Part model, mm, in its own coordinate system. Round coordinates to 2 decimals unless told otherwise and drop trailing zeros. Loops run counter-clockwise (first coordinate to the right, second up) from the corner with the lowest first, then second, coordinate; pieces in that order, holes last. Notation, with made-up numbers: (-5.75, 40) - (14.25, 40) arc R24 cw to (14.25, 51) - close; hole circle Ø9 at (-39, -19). An arc over 180 degrees is marked (long way). Write each question's results on one line, items separated by ' | '. Start each with the question number.
(1) Mould opens along Y. For faces 1 (the face through (45, 0, 1)), 2 (the face through (0, -27, 1)), 3 (the face through (-42.49, 24.13, 0.81)) say: released by +Y, released by -Y, zero draft, split by the parting line, or undercut.
(2) Flat gauge pin, fed straight in: P1, Ø2.5, axis at x = -41.3, y = -24, coming from the +Z side. Where does the tip first touch, or does it go through?
(3) Cut at A-A, the plane y = -24. List the corners of the cut face in (x, z), then the cut area to 3 significant figures.
(4) Drill centre lines: L1, parallel to X at y = -16, z = 0.1; L2, parallel to X at y = 1.5, z = 0.45. Where is each one in solid material? Low to high.
from build123d import *

# Parameters (mm, degrees)
SKIZZE1_W                       = 89.3
SKIZZE1_H                       = 55.04
AUFSATZ_LINEAR_AUSTRAGEN1_DEPTH = 1.6
SKIZZE2_R                       = 1.5
SKIZZE2_R_2                     = 0.5
SCHNITT_LINEAR_AUSTRAGEN1_DEPTH = 1.6


with BuildPart() as part:
    # Skizze1 → Aufsatz-Linear austragen1 (new body)
    with BuildSketch(Plane.XY):
        with Locations((0.35, 0.52)):
            Rectangle(SKIZZE1_W, SKIZZE1_H)
    extrude(amount=AUFSATZ_LINEAR_AUSTRAGEN1_DEPTH)

    # Skizze2 → Schnitt-Linear austragen1 (cut)
    with BuildSketch(Plane.XY.offset(1.6)):
        with Locations((-41.3, 25.04)):
            Circle(SKIZZE2_R)
        with Locations((-41.3, -24)):
            Circle(SKIZZE2_R)
        with Locations((42, 25.04)):
            Circle(SKIZZE2_R)
        with Locations((42, -24)):
            Circle(SKIZZE2_R)
        with Locations((43, 17.03)):
            Circle(SKIZZE2_R_2)
        with Locations((43, 14.49)):
            Circle(SKIZZE2_R_2)
        with Locations((43, 11.95)):
            Circle(SKIZZE2_R_2)
        with Locations((43, 9.41)):
            Circle(SKIZZE2_R_2)
        with Locations((43, 6.87)):
            Circle(SKIZZE2_R_2)
        with Locations((43, 4.33)):
            Circle(SKIZZE2_R_2)
        with Locations((43, 1.79)):
            Circle(SKIZZE2_R_2)
        with Locations((43, -0.75)):
            Circle(SKIZZE2_R_2)
        with Locations((43, -3.29)):
            Circle(SKIZZE2_R_2)
        with Locations((43, -5.83)):
            Circle(SKIZZE2_R_2)
        with Locations((43, -8.37)):
            Circle(SKIZZE2_R_2)
        with Locations((43, -10.91)):
            Circle(SKIZZE2_R_2)
        with Locations((43, -13.45)):
            Circle(SKIZZE2_R_2)
        with Locations((-41.3, 4.33)):
            Circle(SKIZZE2_R_2)
        with Locations((-41.3, 1.79)):
            Circle(SKIZZE2_R_2)
        with Locations((-41.3, -0.75)):
            Circle(SKIZZE2_R_2)
        with Locations((43, -15.99)):
            Circle(SKIZZE2_R_2)
        with Locations((-41.3, -3.29)):
            Circle(SKIZZE2_R_2)
    extrude(amount=-SCHNITT_LINEAR_AUSTRAGEN1_DEPTH, mode=Mode.SUBTRACT)


solid = part.part
A:
1) face 1: zero draft | face 2: released by -Y | face 3: undercut
2) P1: through
3) outline: (-44.3, 0) - (-42.8, 0) - (-42.8, 1.6) - (-44.3, 1.6) - close; (-39.8, 0) - (40.5, 0) - (40.5, 1.6) - (-39.8, 1.6) - close; (43.5, 0) - (45, 0) - (45, 1.6) - (43.5, 1.6) - close | area: 133 mm2
4) L1: -44.3 to 42.5, 43.5 to 45 | L2: -44.3 to -41.71, -40.89 to 42.59, 43.41 to 45
